Autodesk Inventor part; units mm, degrees
ref_plane "YZ Plane" through (0, 0, 0) normal (1, 0, 0) x (0, 1, 0)
ref_plane "XZ Plane" through (0, 0, 0) normal (0, 1, 0) x (-1, 0, 0)
ref_plane "XY Plane" through (0, 0, 0) normal (0, 0, 1) x (1, 0, 0)
sketch "Sketch1" plane through (0, 0, 0) normal (0, 1, 0) x (-1, 0, 0)
  line L0 (-10.16, 10.16) -> (10.16, 10.16)
  line L1 (10.16, 10.16) -> (10.16, -10.16)
  line L2 (10.16, -10.16) -> (-10.16, -10.16)
  line L3 (-10.16, -10.16) -> (-10.16, 10.16)
  circle A0 centre (0, 0) radius 8.255
  dimension "d0" = 20.32
  dimension "d1" = 20.32
  dimension "d2" = 10.16
  dimension "d3" = 10.16
  dimension "d4" = 16.51
extrude "Extrusion1" add sketch "Sketch1" along normal blind 16.51
sketch "Sketch2" plane through (10.16, 0, 10.16) normal (1, 0, 0) x (0, 0, -1)
  line L0 (1.778, 12.446) -> (2.921, 5.08)
  line L1 (2.921, 5.08) -> (17.399, 5.08)
  line L2 (17.399, 5.08) -> (18.542, 12.446)
  line L3 (18.542, 12.446) -> (1.778, 12.446)
  line L4 (20.32, 0) -> (0, 0)
  line L5 (20.32, 0) -> (20.32, 16.51)
  point P0 (10.16, 0)
  dimension "d7" = 16.764
  dimension "d8" = 14.478
  dimension "d9" = 7.366
  dimension "d10" = 5.08
  dimension "d11" = 2.921
extrude "Extrusion2" add sketch "Sketch2" along normal blind 12.7
sketch "Sketch3" plane through (10.16, 12.446, 8.382) normal (0, 1, 0) x (1, 0, 0)
  circle A0 centre (5.842, 8.382) radius 2.286
  line L0 (12.7, 16.764) -> (12.7, 0)
  point P0 (-10.16, 8.382)
  dimension "d14" = 4.572
  dimension "d15" = 6.858
extrude "Extrusion3" cut sketch "Sketch3" against normal blind 17.78
properties part number "HopperFinal1"
CAD build for the part. Positions are in the model's coordinates, mm. A direction names the side the tool comes from. Give positions to 0.01 mm unless a question says otherwise; leave off trailing zeros. Write each loop counter-clockwise with the first axis right and the second up, starting at its lowest first coordinate (ties: lowest second). Pieces come first, ordered by that corner, then holes. Notation, with made-up numbers: (18, -16.75) -> (71, -16.75) arc R29 ccw to (71, 14.25) -> close; hole circle Ø1 at (88, -39.5). An arc over 180 degrees is marked (long way). Return JSON: item names as keys, results as strings.
Item 1: Band-saw the part on B-B (x = 0). List the corners of the cut face in (y, z) (3 decimals).
Answer below:
{"outline": "(0, -10.16) -> (16.51, -10.16) -> (16.51, -8.255) -> (0, -8.255) -> close; (0, 8.255) -> (16.51, 8.255) -> (16.51, 10.16) -> (0, 10.16) -> close"}
Item 2: Drill centre lines: probe 1 along Z at (x, y) = (0, 9) (3 decimals); probe 2 along X at (y, z) = (5.25, 1.5); probe 3 along Z at (x, y) = (17.5, 9.75). Where is each one in solid material? Low to high.
Answer below:
{"probe 1": "z = -10.16 to -8.255, 8.255 to 10.16", "probe 2": "x = -10.16 to -8.12, 8.12 to 14.28, 17.73 to 22.86", "probe 3": "z = -7.96 to -1.73, 1.73 to 7.96"}
Item 3: Band-saw the part on A-A (z = 0). List the corners of the cut face in (x, y) (3 decimals).
Answer below:
{"outline": "(-10.16, 0) -> (-8.255, 0) -> (-8.255, 16.51) -> (-10.16, 16.51) -> close; (8.255, 0) -> (10.16, 0) -> (10.16, 5.08) -> (13.716, 5.08) -> (13.716, 12.446) -> (10.16, 12.446) -> (10.16, 16.51) -> (8.255, 16.51) -> close; (18.288, 5.08) -> (22.86, 5.08) -> (22.86, 12.446) -> (18.288, 12.446) -> close"}
Item 4: Band-saw the part on C-C (y = 2). List the corners of the cut face in (x, z) (3 decimals).
Answer below:
{"outline": "(-10.16, -10.16) -> (10.16, -10.16) -> (10.16, 10.16) -> (-10.16, 10.16) -> close; hole circle Ø16.51 at (0, 0)"}
Item 5: Band-saw the part on D-D (z = -6.25). List the corners of the cut face in (x, y).
Answer below:
{"outline": "(-10.16, 0) -> (-5.39, 0) -> (-5.39, 16.51) -> (-10.16, 16.51) -> close; (5.39, 0) -> (10.16, 0) -> (10.16, 5.08) -> (22.86, 5.08) -> (22.86, 12.45) -> (10.16, 12.45) -> (10.16, 16.51) -> (5.39, 16.51) -> close"}
Item 6: Two-plate mould, pull along X, no slides. Class faces 6 (the cylindrical face through (18.11, 8.81, 0.88)), 7 (the flat face through (5, 16.51, 7)), 8 (the flat face through (22.86, 9, 0)): +X half, -X half, draft (parallel to the pull), parting line (faces both ways), or undercut.
Answer below:
{"face 6": "undercut", "face 7": "draft", "face 8": "+X half"}
Item 7: Tool access for faces 1 (the flat face through (16.4, 8.7, -7.8)), 2 (the flat face through (18, 5.08, 2)), 3 (the cylindrical face through (-7.874, 8.139, -2.48)), 4 (the flat face through (16.421, 8.815, 7.819)), 5 (the flat face through (18, 12.446, -2)): list every direction of +Z, -Z, +X, -X, +Y, -Y with a clear straight run to the whole face (end or side of a thin tool).
Answer below:
{"face 1": "-Z, +X, -Y", "face 2": "+Z, -Z, +X, -Y", "face 3": "+Y, -Y", "face 4": "+Z, +X, -Y", "face 5": "+Z, -Z, +X, +Y"}
Item 8: Drop flat-ended pins along their axis: pin 1 (3 mm diameter, centred on x = 14, z = 7.5, fed in from +Y); pin 2 (8 mm diameter, centred on x = 14.5, z = 0.5, fed in from -Y). Give the stop position or say it passes through.
Answer below:
{"pin 1": "stops at y = 12.45", "pin 2": "stops at y = 5.08"}
